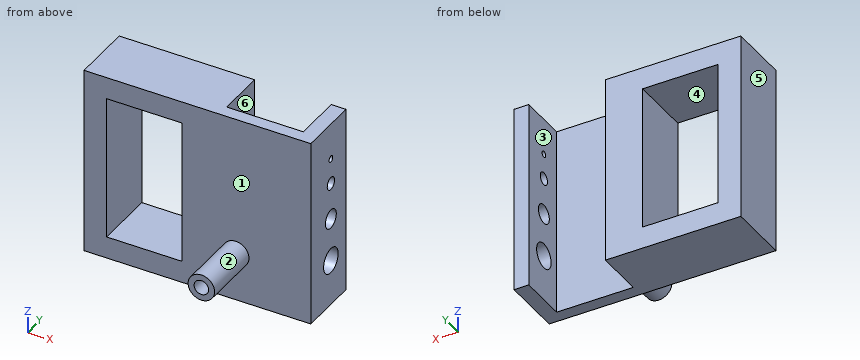
from build123d import *

# Parameters (mm, degrees)
SKETCH_1_W          = 36
SKETCH_1_H          = 30
SKETCH_1_W_2        = 12
SKETCH_1_H_2        = 23
EXTRUDE_1_DEPTH     = 10
SKETCH_1_4_R        = 2.55
EXTRUDE_2_DEPTH     = 6
SKETCH_2_W          = 12.160825217
SKETCH_2_H          = 34.685599871
CUT_EXTRUDE_1_DEPTH = 8
SKETCH_3_R          = 0.5
SKETCH_3_R_2        = 1
SKETCH_3_R_3        = 1.5
SKETCH_3_R_4        = 2
CUT_EXTRUDE_2_DEPTH = 8
SKETCH_4_R          = 4.417962551
CUT_EXTRUDE_3_DEPTH = 0.1
SKETCH_5_R          = 5.05323065
CUT_EXTRUDE_4_DEPTH = 1.4
SKETCH_6_R          = 1
CUT_EXTRUDE_6_DEPTH = 10
SKETCH_11_R         = 2.55
SKETCH_11_R_2       = 1
EXTRUDE_3_DEPTH     = 5
SKETCH_12_OUTSIDE_W = 48.152
SKETCH_12_OUTSIDE_H = 42.152
SKETCH_12_OUTSIDE_R = 2.1
CUT_EXTRUDE_7_DEPTH = 9.5
SKETCH_13_R         = 1.15
CUT_EXTRUDE_8_DEPTH = 13.5
SKETCH_14_W         = 102.67858786
SKETCH_14_H         = 80.280273631
CUT_EXTRUDE_9_DEPTH = 0.3


with BuildPart() as part:
    # Sketch 1 → Extrude 1 (new body)
    with BuildSketch(Plane(origin=(0, 0, 0), x_dir=(1, 0, 0), z_dir=(0, 1, 0))):
        Rectangle(SKETCH_1_W, SKETCH_1_H)
        with Locations((-8.41025641, 0)):
            Rectangle(SKETCH_1_W_2, SKETCH_1_H_2, mode=Mode.SUBTRACT)
    extrude(amount=EXTRUDE_1_DEPTH)

    # Sketch 1_4 → Extrude 2 (add)
    with BuildSketch(Plane(origin=(0, 0, 0), x_dir=(1, 0, 0), z_dir=(0, 1, 0))):
        with Locations(Location((6.08974359, 7.376281108, 0), (0, 0, 270))):
            Circle(SKETCH_1_4_R)
    extrude(amount=-EXTRUDE_2_DEPTH)

    # Sketch 2 → Cut-Extrude 1 (cut)
    with BuildSketch(Plane(origin=(0, 10, 0), x_dir=(1, 0, 0), z_dir=(0, 1, 0))):
        with Locations((9.579402218, 0.667301742)):
            Rectangle(SKETCH_2_W, SKETCH_2_H)
    extrude(amount=-CUT_EXTRUDE_1_DEPTH, mode=Mode.SUBTRACT)

    # Sketch 3 → Cut-Extrude 2 (cut)
    with BuildSketch(Plane(origin=(18, 0, 0), x_dir=(0, 0, -1), z_dir=(1, 0, 0))):
        with Locations((-9.184219858, 5.534894538)):
            Circle(SKETCH_3_R)
        with Locations((-5.107163581, 5.534894538)):
            Circle(SKETCH_3_R_2)
        with Locations((0.769869669, 5.534894538)):
            Circle(SKETCH_3_R_3)
        with Locations((7.709539928, 5.534894538)):
            Circle(SKETCH_3_R_4)
    extrude(amount=-CUT_EXTRUDE_2_DEPTH, mode=Mode.SUBTRACT)

    # Sketch 4 → Cut-Extrude 3 (cut)
    with BuildSketch(Plane.XZ.offset(6)):
        with Locations((5.795390071, -7.128470111)):
            Circle(SKETCH_4_R)
    extrude(amount=-CUT_EXTRUDE_3_DEPTH, mode=Mode.SUBTRACT)

    # Sketch 5 → Cut-Extrude 4 (cut)
    with BuildSketch(Plane.XZ.offset(5.9)):
        with Locations((5.767325228, -7.296859169)):
            Circle(SKETCH_5_R)
    extrude(amount=-CUT_EXTRUDE_4_DEPTH, mode=Mode.SUBTRACT)

    # Sketch 6 → Cut-Extrude 6 (cut)
    with BuildSketch(Plane.XZ.offset(4.5)):
        with Locations(Location((6.08974359, -7.376281108, 0), (0, 0, 270))):
            Circle(SKETCH_6_R)
    extrude(amount=-CUT_EXTRUDE_6_DEPTH, mode=Mode.SUBTRACT)

    # Sketch 11 → Extrude 3 (add)
    with BuildSketch(Plane.XZ.offset(4.5)):
        with Locations(Location((6.08974359, -7.376281108, 0), (0, 0, 90))):
            Circle(SKETCH_11_R)
        with Locations(Location((6.08974359, -7.376281108, 0), (0, 0, 270))):
            Circle(SKETCH_11_R_2, mode=Mode.SUBTRACT)
    extrude(amount=EXTRUDE_3_DEPTH)

    # Sketch 12 outside → Cut-Extrude 7 (cut)
    with BuildSketch(Plane.XZ.offset(9.5)):
        Rectangle(SKETCH_12_OUTSIDE_W, SKETCH_12_OUTSIDE_H)
        with Locations(Location((6.08974359, -7.376281108, 0), (0, 0, 270))):
            Circle(SKETCH_12_OUTSIDE_R, mode=Mode.SUBTRACT)
    extrude(amount=-CUT_EXTRUDE_7_DEPTH, mode=Mode.SUBTRACT)

    # Sketch 13 → Cut-Extrude 8 (cut)
    with BuildSketch(Plane.XZ.offset(9.5)):
        with Locations(Location((6.08974359, -7.376281108, 0), (0, 0, 270))):
            Circle(SKETCH_13_R)
    extrude(amount=-CUT_EXTRUDE_8_DEPTH, mode=Mode.SUBTRACT)

    # Sketch 14 → Cut-Extrude 9 (cut)
    with BuildSketch(Plane(origin=(0, 10, 0), x_dir=(1, 0, 0), z_dir=(0, 1, 0))):
        with Locations((-27.117967051, 18.219550081)):
            Rectangle(SKETCH_14_W, SKETCH_14_H)
    extrude(amount=-CUT_EXTRUDE_9_DEPTH, mode=Mode.SUBTRACT)


solid = part.part
The model under review builds one solid part; all positions refer to its coordinate system, in mm. Face numbers are marked on the shaded views. A direction names the side the tool comes from. Give positions to 0.01 mm unless a question says otherwise; leave off trailing zeros. Write each loop counter-clockwise with the first axis right and the second up, starting at its lowest first coordinate (ties: lowest second). Pieces come first, ordered by that corner, then holes. Notation, with made-up numbers: M 6,2.25 L 19,2.25 A11 cw 19,17.25 Z; hole C 34,43 d9. An arc over 180 degrees is marked long. One line per question, with ' | ' between items. Start each with the question number.
Item 1: We need section B-B on x = -3. Write out the cut boundary in (y, z).
Item 2: Draft analysis for pull direction X (two halves, no side actions). For the marked faces 1, 2 and 3, state which applies: released by +X, released by -X, zero draft, split by the parting line, or undercut.
Item 3: We need section D-D on z = 12.75. Write out the cut boundary in (x, y).
Item 4: Wall thickness on line 1 (X direction, y = 4, z = 1.75); line 2 (X direction, y = 2.5, z = -13); line 3 (Z direction, x = -8.5, y = 3): over which ranges is each line inside the solid? List them lowest first. Write a range as from..to.
Item 5: We need section A-A on y = 2.75. Write out the cut boundary in (x, z), plus the area to 3 significant figures.
Item 6: For pin 1 (12 mm diameter, centred on x = 3.5, z = -2, fed in from -Y); pin 2 (8 mm diameter, centred on x = -1.5, z = -1.5, fed in from -Y); pin 3 (3.5 mm diameter, centred on x = 6.09, z = -7.38, fed in from +Y), all flat-tipped, find the tip position at first contact; note any pin that passes through.
Item 7: For the marked faces 4, 5 and 6, list the 3-axis set-ups (+Z, -Z, +X, -X, +Y, -Y) from which the entire face can be reached by the end or side of a thin tool; tool diameter is ignored.
Item 8: We need section C-C on z = -4.25. Write out the cut boundary in (x, y), plus the area to 3 significant figures.
Results found:
1) outline: M 0,-15 L 9.7,-15 L 9.7,-11.5 L 0,-11.5 Z; M 0,11.5 L 9.7,11.5 L 9.7,15 L 0,15 Z
2) face 1: zero draft | face 2: split by the parting line | face 3: undercut
3) outline: M -18,0 L 18,0 L 18,9.7 L 15.66,9.7 L 15.66,2 L 3.5,2 L 3.5,9.7 L -18,9.7 Z
4) line 1: x = -18..-14.41, -2.41..3.5, 15.66..18 | line 2: x = -18..3.5, 15.66..18 | line 3: z = -15..-11.5, 11.5..15
5) outline: M -18,-15 L 3.5,-15 L 3.5,15 L -18,15 Z; M 15.66,-15 L 18,-15 L 18,15 L 15.66,15 Z; hole M -14.41,-11.5 L -2.41,-11.5 L -2.41,11.5 L -14.41,11.5 Z | area: 439 mm2
6) pin 1: stops at y = -9.5 | pin 2: stops at y = 0 | pin 3: stops at y = 2
7) face 4: +Y, -Y | face 5: +Z, -Z, -X, +Y, -Y | face 6: +Z, -Z, +Y
8) outline: M -18,0 L -14.41,0 L -14.41,9.7 L -18,9.7 Z; M -2.41,0 L 18,0 L 18,9.7 L 15.66,9.7 L 15.66,2 L 3.5,2 L 3.5,9.7 L -2.41,9.7 Z | area: 139 mm2
